Build history of the part. All positions in model axes, mm. A direction names the side the tool comes from. Give positions to 0.01 mm unless a question says otherwise; leave off trailing zeros. Write each loop counter-clockwise with the first axis right and the second up, starting at its lowest first coordinate (ties: lowest second). Pieces come first, ordered by that corner, then holes.
Autodesk Inventor part; units mm, degrees
ref_plane "YZ Plane" through (0, 0, 0) normal (1, 0, 0) x (0, 1, 0)
ref_plane "XZ Plane" through (0, 0, 0) normal (0, 1, 0) x (-1, 0, 0)
ref_plane "XY Plane" through (0, 0, 0) normal (0, 0, 1) x (1, 0, 0)
sketch "Sketch1" plane through (0, 0, 0) normal (0, 1, 0) x (-1, 0, 0)
  line L0 (0, 0) -> (0, -312.648) construction
  line L1 (5, 0) -> (5, -312.648)
  line L2 (-5, -312.648) -> (-5, 0)
  arc A0 (5, 0) -> (-5, 0) centre (0, 0) ccw
  arc A1 (-5, -312.648) -> (5, -312.648) centre (0, -312.648) ccw
  circle A2 centre (0, 0) radius 1.65
  circle A3 centre (0, -312.648) radius 1.65
  circle A4 centre (0, -42.6) radius 1.65
  circle A5 centre (0, -254.274) radius 1.65
  arc A6 (5, -254.274) -> (5, -42.6) centre (-585.5917, -148.437) ccw
  arc A7 (-5, -254.274) -> (-5, -42.6) centre (-595.5917, -148.437) ccw
  circle A8 centre (7.5096, -100) radius 1.65
  point P0 (0, -156.324)
  dimension "d0" = 3.3
  dimension "d1" = 3.3
  dimension "d2" = 10
  dimension "d3" = 312.648
  dimension "d10" = 3.3
  dimension "d11" = 42.6
  dimension "d12" = 3.3
  dimension "d13" = 254.274
  dimension "d16" = 600
  dimension "d17" = 600
  dimension "d18" = 3.3
  dimension "d19" = 100
extrude "Extrusion1" add sketch "Sketch1" along normal blind 6 contours L1 A1 L2 A7 A0 | A6 L1
sketch "Sketch2" plane through (0, 6, 0) normal (0, 1, 0) x (1, 0, 0)
  line L0 (-42.2974, 163.7654) -> (39.2104, 163.7654)
  line L1 (39.2104, 163.7654) -> (39.2104, -15.6831)
  line L2 (39.2104, -15.6831) -> (-42.2974, -15.6831)
  line L3 (-42.2974, -15.6831) -> (-42.2974, 163.7654)
  line L4 (-108.6868, 337.298) -> (118.0888, 337.298)
  line L5 (118.0888, 337.298) -> (118.0888, -100.4775)
  line L6 (118.0888, -100.4775) -> (-108.6868, -100.4775)
  line L7 (-108.6868, -100.4775) -> (-108.6868, 337.298)
  point P0 (0, 0)
extrude "Extrusion2" cut sketch "Sketch2" against normal blind 10
properties part number "Part_16_p1"
1. Drop flat-ended pins along their axis: pin 1 (1 mm diameter, centred on y = 2, z = -96, fed in from -X); pin 2 (1.8 mm diameter, centred on y = 2, z = -17, fed in from -X); pin 3 (3 mm diameter, centred on x = 0, z = -42.6, fed in from +Y). Give the stop position or say it passes through.
2. Mould opens along X. For faces 4 (the face through (-12.616, 2.958, -102.099)), 5 (the face through (-0.89, 2.96, -43.99)), 6 (the face through (0, 3, 5)), 7 (the face through (-7.15, 2.96, -98.39)) say: pulls with the +X half, pulls with the -X half, needs draft (parallel to the pull), parting line crosses it, or undercut.
3. Drill centre lines: line 1 along X through (y, z) = (3.9, -39); line 2 along X through (y, z) = (1.65, -100); line 3 along X through (y, z) = (5.3, -70). Where is each one in solid material? Low to high.
4. Saw through at B-B on y = 3.5. Give the cut face in (x, z).
5. 3-axis set-ups, long thin cutter, end or side, ignore diameter. For faces 1 (the face through (-5, 3, -21)), 2 (the face through (-2.616, 2.958, -102.099)), 3 (the face through (-9, 3, -163.765)): which of +Z, -Z, +X, -X, +Y, -Y reach the whole face in a straight line?
6. Saw through at A-A on z = -100. Give the cut face in (x, y).
7. Saw through at C-C on x = 0. Give the cut face in (y, z).
8. Saw through at D-D on z = -75. Give the cut face in (x, y), plus the area to 3 significant figures.
Outcome:
1. pin 1: stops at x = -12.16
1. pin 2: stops at x = -5
1. pin 3: passes through
2. face 4: pulls with the -X half
2. face 5: undercut
2. face 6: parting line crosses it
2. face 7: undercut
3. line 1: x = -5 to 5
3. line 2: x = -12.45 to -9.16, -5.86 to -2.45
3. line 3: x = -9.26 to 0.74
4. outline: (-14.21, -163.77) - (-4.21, -163.77) arc R600 cw to (5, -42.6) - (5, 0) arc R5 ccw to (-5, 0) - (-5, -42.6) arc R600 ccw to start; hole circle Ø3.3 at (-7.51, -100); hole circle Ø3.3 at (0, -42.6); hole circle Ø3.3 at (0, 0)
5. face 1: +Z, -X, +Y, -Y
5. face 2: +X, +Y, -Y
5. face 3: -Z, +X, -X, +Y, -Y
6. outline: (-12.45, 0) - (-9.16, 0) - (-9.16, 6) - (-12.45, 6) - close; (-5.86, 0) - (-2.45, 0) - (-2.45, 6) - (-5.86, 6) - close
7. outline: (0, -75.84) - (6, -75.84) - (6, -44.25) - (0, -44.25) - close; (0, -40.95) - (6, -40.95) - (6, -1.65) - (0, -1.65) - close; (0, 1.65) - (6, 1.65) - (6, 5) - (0, 5) - close
8. outline: (-9.9, 0) - (0.1, 0) - (0.1, 6) - (-9.9, 6) - close
8. area: 60.0 mm2
